Part model, mm, in its own coordinate system. A direction names the side the tool comes from. Round coordinates to 2 decimals unless told otherwise and drop trailing zeros. Write each loop counter-clockwise with the first axis right and the second up, starting at its lowest first coordinate (ties: lowest second). Pieces come first, ordered by that corner, then holes. Notation, with made-up numbers: (63, -26.75) -> (79, -26.75) arc R22 ccw to (79, -2.75) -> close; hole circle Ø2 at (35, 88.25). An arc over 180 degrees is marked (long way). Return JSON: item names as keys, results as strings. Group by question number.
(1) Tool access for faces 4 (the cylindrical face through (3.47, 15.62, 3.14)), 5 (the cylindrical face through (3.306, 14.887, 35.439)): list every direction of +Z, -Z, +X, -X, +Y, -Y with a clear straight run to the whole face (end or side of a thin tool).
(2) Drop flat-ended pins along their axis: pin 1 Ø3 at (y, z) = (-4, 22.5) entering from -X; pin 2 Ø8 at (y, z) = (-11, 28.5) entering from -X; pin 3 Ø5 at (y, z) = (5, 31) entering from +X. Give the stop position or say it passes through.
(3) Mould opens along Z. For faces 1 (the cylindrical face through (3.306, 14.887, 6.539)), 2 (the flat face through (-4, 14, 42)), 3 (the cylindrical face through (3.47, 15.62, 38.79)) say: +Z half, -Z half, draft (parallel to the pull), parting line (faces both ways), or undercut.
(4) Drill centre lines: L1, parallel to Y at x = 0, z = 27; L2, parallel to X at y = -0.5, z = 2.5; L3, parallel to Y at x = -13, z = 38.5. Where is each one in solid material? Low to high. Write a range as from..to.
(5) Saw through at C-C (z = 5). List the corners of the cut face in (x, y), plus the area to 3 significant figures.
(6) Saw through at A-A (y = 0). List the corners of the cut face in (x, z), plus the area to 3 significant figures.
from build123d import *

# Parameters (mm, degrees)
SKETCH1_R           = 16
SKETCH1_R_2         = 14.3
BOSS_EXTRUDE1_DEPTH = 42
SKETCH3_W           = 0.75
SKETCH3_H           = 1.6
FILLET1_R           = 0.6


with BuildPart() as part:
    # Sketch1 → Boss-Extrude1 (new body)
    with BuildSketch(Plane.XY):
        with Locations(Location((0, 0, 0), (0, 0, 180))):
            Circle(SKETCH1_R)
        with Locations(Location((0, 0, 0), (0, 0, 180))):
            Circle(SKETCH1_R_2, mode=Mode.SUBTRACT)
    extrude(amount=BOSS_EXTRUDE1_DEPTH)

    # Sketch3 → Cut-Revolve2 (revolve, cut)
    with BuildSketch(Plane(origin=(0, 0, 0), x_dir=(1, 0, 0), z_dir=(0, 1, 0)), mode=Mode.PRIVATE) as cut_revolve2_sk:
        with Locations((15.625, -35.45)):
            Rectangle(SKETCH3_W, SKETCH3_H)
        with Locations((15.625, -6.55)):
            Rectangle(SKETCH3_W, SKETCH3_H)
    revolve(cut_revolve2_sk.sketch.rotate(Axis((0, 0, 0), (0, 0, 1)), 180), axis=Axis((0, 0, 0), (0, 0, 1)), mode=Mode.SUBTRACT)

    # Fillet1
    fillet1_edges = [part.edges().sort_by_distance(p)[0] for p in [
        (16, 0, 0),
        (16, 0, 42),
    ]]
    fillet(fillet1_edges, radius=FILLET1_R)


solid = part.part
Computed values:
{
 "1": {"face 4": "+Z, -Z", "face 5": "none"},
 "2": {"pin 1": "x = -15.8", "pin 2": "x = -14.39", "pin 3": "x = 15.8"},
 "3": {"face 1": "undercut", "face 2": "+Z half", "face 3": "draft"},
 "4": {"L1": "-16..-14.3, 14.3..16", "L2": "-15.99..-14.29, 14.29..15.99", "L3": "-9.33..-5.96, 5.96..9.33"},
 "5": {"outline": "circle Ø32 at (0, 0); hole circle Ø28.6 at (0, 0)", "area": "162 mm2"},
 "6": {"outline": "(-16, 0.6) arc R0.6 ccw to (-15.4, 0) -> (-14.3, 0) -> (-14.3, 42) -> (-15.4, 42) arc R0.6 ccw to (-16, 41.4) -> (-16, 36.25) -> (-15.25, 36.25) -> (-15.25, 34.65) -> (-16, 34.65) -> (-16, 7.35) -> (-15.25, 7.35) -> (-15.25, 5.75) -> (-16, 5.75) -> close; (14.3, 0) -> (15.4, 0) arc R0.6 ccw to (16, 0.6) -> (16, 5.75) -> (15.25, 5.75) -> (15.25, 7.35) -> (16, 7.35) -> (16, 34.65) -> (15.25, 34.65) -> (15.25, 36.25) -> (16, 36.25) -> (16, 41.4) arc R0.6 ccw to (15.4, 42) -> (14.3, 42) -> close", "area": "138 mm2"}
}
